from build123d import *

# Parameters (mm, degrees)
F0_R     = 11.2
F1_DEPTH = 7


with BuildPart() as f1:
    # F0 (on Top) → F1 (new body)
    with BuildSketch(Plane.XY):
        with BuildLine():
            Line((-21.939748, 4.555207), (-12.792678, 3.253825))
            ThreePointArc((-12.792678, 3.253825), (-11.283485, -6.850034), (-3.015751, -12.850885))
            Line((-3.015751, -12.850885), (-7.8557, -22.943517))
            Line((-7.8557, -22.943517), (-9.711457, -26.813285))
            Line((-9.711457, -26.813285), (-11.121781, -27.627536))
            Line((-11.121781, -27.627536), (-20.063522, -32.790052))
            Line((-20.063522, -32.790052), (-27.45722, -32.629778))
            Line((-27.45722, -32.629778), (-35.012019, -31.040825))
            Line((-35.012019, -31.040825), (-33.880058, -33.001439))
            Line((-33.880058, -33.001439), (-26.171613, -34.856514))
            Line((-26.171613, -34.856514), (-18.97682, -34.672275))
            Line((-18.97682, -34.672275), (-7.830637, -28.237023))
            Line((-7.830637, -28.237023), (-6.368866, -27.393069))
            Line((-6.368866, -27.393069), (-4.491412, -23.347324))
            Line((-4.491412, -23.347324), (0.218357, -13.198194))
            Line((0.218357, -13.198194), (3.914865, -22.392298))
            Line((3.914865, -22.392298), (5.384581, -26.047835))
            Line((5.384581, -26.047835), (6.257514, -26.551823))
            Line((6.257514, -26.551823), (18.746148, -33.762139))
            Line((18.746148, -33.762139), (24.941822, -34.300735))
            Line((24.941822, -34.300735), (33.179322, -33.454726))
            Line((33.179322, -33.454726), (34.46769, -31.223206))
            Line((34.46769, -31.223206), (26.169356, -32.174584))
            Line((26.169356, -32.174584), (19.596018, -31.214334))
            Line((19.596018, -31.214334), (9.226481, -25.227478))
            Line((9.226481, -25.227478), (8.427354, -24.766103))
            Line((8.427354, -24.766103), (7.024949, -21.277983))
            Line((7.024949, -21.277983), (3.578444, -12.705697))
            ThreePointArc((3.578444, -12.705697), (11.574046, -6.346768), (12.637068, 3.813725))
            Line((12.637068, 3.813725), (23.797519, 4.668523))
            Line((23.797519, 4.668523), (28.076715, 4.996274))
            Line((28.076715, 4.996274), (29.487039, 4.182023))
            Line((29.487039, 4.182023), (38.428779, -0.980493))
            Line((38.428779, -0.980493), (41.986827, -7.46376))
            Line((41.986827, -7.46376), (44.388153, -14.800885))
            Line((44.388153, -14.800885), (45.520113, -12.840272))
            Line((45.520113, -12.840272), (43.272433, -5.237025))
            Line((43.272433, -5.237025), (39.515481, 0.901729))
            Line((39.515481, 0.901729), (28.369297, 7.336981))
            Line((28.369297, 7.336981), (26.907526, 8.180935))
            Line((26.907526, 8.180935), (22.465082, 7.783985))
            Line((22.465082, 7.783985), (11.320793, 6.788199))
            Line((11.320793, 6.788199), (17.434867, 14.586522))
            Line((17.434867, 14.586522), (19.865796, 17.687101))
            Line((19.865796, 17.687101), (19.865796, 18.695077))
            Line((19.865796, 18.695077), (19.865796, 33.11571))
            Line((19.865796, 33.11571), (17.234397, 38.750619))
            Line((17.234397, 38.750619), (12.382981, 45.461498))
            Line((12.382981, 45.461498), (9.806245, 45.461498))
            Line((9.806245, 45.461498), (14.77933, 38.750619))
            Line((14.77933, 38.750619), (17.234397, 32.577816))
            Line((17.234397, 32.577816), (17.234397, 20.604106))
            Line((17.234397, 20.604106), (17.234397, 19.681354))
            Line((17.234397, 19.681354), (14.9148, 16.722776))
            Line((14.9148, 16.722776), (9.214235, 9.451872))
            ThreePointArc((9.214235, 9.451872), (-0.290561, 13.196802), (-9.621317, 9.03716))
            Line((-9.621317, 9.03716), (-15.941819, 18.274994))
            Line((-15.941819, 18.274994), (-18.365257, 21.817012))
            Line((-18.365257, 21.817012), (-18.365257, 23.445513))
            Line((-18.365257, 23.445513), (-18.365257, 33.770546))
            Line((-18.365257, 33.770546), (-14.529607, 40.093539))
            Line((-14.529607, 40.093539), (-9.376134, 45.84171))
            Line((-9.376134, 45.84171), (-11.640055, 45.84171))
            Line((-11.640055, 45.84171), (-17.10082, 40.093539))
            Line((-17.10082, 40.093539), (-20.538661, 33.770546))
            Line((-20.538661, 33.770546), (-20.538661, 20.900042))
            Line((-20.538661, 20.900042), (-20.538661, 19.212134))
            Line((-20.538661, 19.212134), (-17.97367, 15.563339))
            Line((-17.97367, 15.563339), (-11.53915, 6.409994))
            Line((-11.53915, 6.409994), (-21.349732, 7.805776))
            Line((-21.349732, 7.805776), (-25.250377, 8.360733))
            Line((-25.250377, 8.360733), (-26.12331, 7.856745))
            Line((-26.12331, 7.856745), (-38.611944, 0.646429))
            Line((-38.611944, 0.646429), (-42.176219, -4.449884))
            Line((-42.176219, -4.449884), (-45.562303, -12.006773))
            Line((-45.562303, -12.006773), (-44.273935, -14.238292))
            Line((-44.273935, -14.238292), (-40.948685, -6.576035))
            Line((-40.948685, -6.576035), (-36.830415, -1.363483))
            Line((-36.830415, -1.363483), (-26.460878, 4.623372))
            Line((-26.460878, 4.623372), (-25.661751, 5.084748))
            Line((-25.661751, 5.084748), (-21.939748, 4.555207))
        make_face()
        Circle(F0_R, mode=Mode.SUBTRACT)
        with BuildLine():
            Line((-9.711457, -26.813285), (-7.8557, -22.943517))
            ThreePointArc((-7.8557, -22.943517), (-12.025565, -21.787106), (-15.940622, -19.943903))
            ThreePointArc((-15.940622, -19.943903), (-16.27639, -12.118209), (-20.987711, -5.860599))
            ThreePointArc((-20.987711, -5.860599), (-23.219885, -4.563891), (-25.661751, -3.726428))
            ThreePointArc((-25.661751, -3.726428), (-41.175768, -20.890944), (-18.369131, -24.78487))
            ThreePointArc((-18.369131, -24.78487), (-14.840432, -26.448342), (-11.121781, -27.627536))
            Line((-11.121781, -27.627536), (-9.711457, -26.813285))
        make_face()
        with Locations((-28.702531, -16.571414)):
            Circle(F0_R, mode=Mode.SUBTRACT)
        with BuildLine():
            Line((-6.368866, -27.393069), (-7.830637, -28.237023))
            ThreePointArc((-7.830637, -28.237023), (-0.682852, -28.261424), (6.257514, -26.551823))
            Line((6.257514, -26.551823), (5.384581, -26.047835))
            Line((5.384581, -26.047835), (3.914865, -22.392298))
            ThreePointArc((3.914865, -22.392298), (-0.248488, -23.220008), (-4.491412, -23.347324))
            Line((-4.491412, -23.347324), (-6.368866, -27.393069))
        make_face()
        with BuildLine():
            Line((8.427354, -24.766103), (9.226481, -25.227478))
            ThreePointArc((9.226481, -25.227478), (12.8176, -23.040102), (16.058057, -20.360514))
            ThreePointArc((16.058057, -20.360514), (38.679972, -25.213789), (30.648892, -3.515699))
            ThreePointArc((30.648892, -3.515699), (30.325152, 0.37198), (29.487039, 4.182023))
            Line((29.487039, 4.182023), (28.076715, 4.996274))
            Line((28.076715, 4.996274), (23.797519, 4.668523))
            ThreePointArc((23.797519, 4.668523), (24.88097, 0.479108), (25.242237, -3.833032))
            ThreePointArc((25.242237, -3.833032), (18.632872, -8.036663), (15.569283, -15.245592))
            ThreePointArc((15.569283, -15.245592), (11.608949, -18.703471), (7.024949, -21.277983))
            Line((7.024949, -21.277983), (8.427354, -24.766103))
        make_face()
        with Locations((28.702531, -16.571414)):
            Circle(F0_R, mode=Mode.SUBTRACT)
        with BuildLine():
            ThreePointArc((28.369297, 7.336981), (24.816537, 13.539344), (19.865796, 18.695077))
            Line((19.865796, 18.695077), (19.865796, 17.687101))
            Line((19.865796, 17.687101), (17.434867, 14.586522))
            ThreePointArc((17.434867, 14.586522), (20.233361, 11.394807), (22.465082, 7.783985))
            Line((22.465082, 7.783985), (26.907526, 8.180935))
            Line((26.907526, 8.180935), (28.369297, 7.336981))
        make_face()
        with BuildLine():
            ThreePointArc((-12.279761, 28.300569), (-15.48472, 26.076362), (-18.365257, 23.445513))
            Line((-18.365257, 23.445513), (-18.365257, 21.817012))
            Line((-18.365257, 21.817012), (-15.941819, 18.274994))
            ThreePointArc((-15.941819, 18.274994), (-12.855404, 21.307998), (-9.301616, 23.776935))
            ThreePointArc((-9.301616, 23.776935), (-2.356482, 20.154872), (5.418428, 21.10619))
            ThreePointArc((5.418428, 21.10619), (10.393206, 19.40538), (14.9148, 16.722776))
            Line((14.9148, 16.722776), (17.234397, 19.681354))
            Line((17.234397, 19.681354), (17.234397, 20.604106))
            ThreePointArc((17.234397, 20.604106), (13.544514, 22.620419), (9.603694, 24.086942))
            ThreePointArc((9.603694, 24.086942), (2.495796, 46.104733), (-12.279761, 28.300569))
        make_face()
        with Locations((0, 33.142827)):
            Circle(F0_R, mode=Mode.SUBTRACT)
        with BuildLine():
            ThreePointArc((-20.538661, 20.900042), (-24.133685, 14.722079), (-26.12331, 7.856745))
            Line((-26.12331, 7.856745), (-25.250377, 8.360733))
            Line((-25.250377, 8.360733), (-21.349732, 7.805776))
            ThreePointArc((-21.349732, 7.805776), (-19.984873, 11.825201), (-17.97367, 15.563339))
            Line((-17.97367, 15.563339), (-20.538661, 19.212134))
            Line((-20.538661, 19.212134), (-20.538661, 20.900042))
        make_face()
        with BuildLine():
            ThreePointArc((-20.987711, -5.860599), (-22.002156, -0.701909), (-21.939748, 4.555207))
            Line((-21.939748, 4.555207), (-25.661751, 5.084748))
            Line((-25.661751, 5.084748), (-26.460878, 4.623372))
            ThreePointArc((-26.460878, 4.623372), (-26.362114, 0.419684), (-25.661751, -3.726428))
            ThreePointArc((-25.661751, -3.726428), (-23.219885, -4.563891), (-20.987711, -5.860599))
        make_face()
    extrude(amount=F1_DEPTH)


solid = f1.part
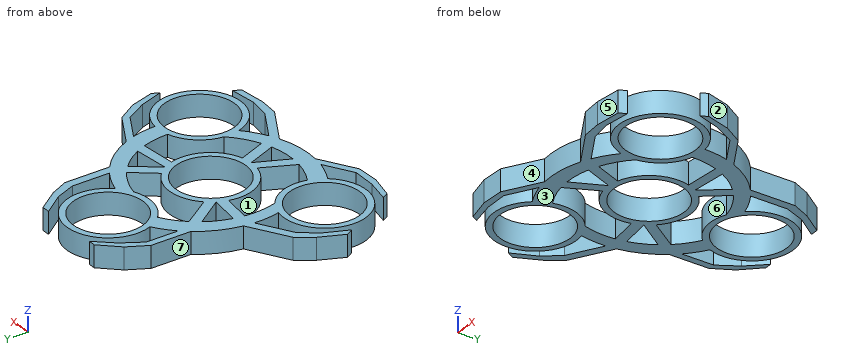
Could you check a few things on this model? Use its own coordinates, in mm. Face numbers are marked on the shaded views. A direction names the side the tool comes from. Coordinates: 2 decimals unless noted, no trailing zeros. Order: outer loops, then holes, each group sorted by start corner. A loop starts at its lowest first (then second) coordinate and runs counter-clockwise, first axis right, second up. Notation, with made-up numbers: (45.25, -17.75) - (54.25, -17.75) arc R9 ccw to (54.25, -7.75) - close; hole circle Ø8 at (47.5, -2). An arc over 180 degrees is marked (long way). Answer in a Markdown table with one row per item. Add a question column.
(1) I need wall thicknesses on L1, parallel to Y at x = -1.5, z = 4.75; L2, parallel to X at y = 34, z = 2.5; L3, parallel to Y at x = -12, z = 5. Which ranges of each line are inside material? Lowest first, please.
(2) On a 3-axis mill with a long thin cutter (end or side, diameter ignored), from which of +Z, -Z, +X, -X, +Y, -Y can I reach the whole of each face in a straight line? I mean the marked faces 4, 5, 6 and 7. Say none if no direction works.
(3) If we mould it in two halves opening along X, with no side actions, what happens to the marked faces 1, 2 and 3? For each: released by +X, released by -X, zero draft, split by the parting line, or undercut.
(4) If we section it at B-B, the plane x = -1: Please give me the cut outline in (y, z).
(5) If we section it at C-C, the plane z = 1: State how many separate pieces and enclosed holes the cut face has, then the cut area to 3 significant figures.
(6) Will these pins go through, and if not, where does the flat tip stop? pin 1 (2 mm diameter, centred on y = 25.5, z = 5, fed in from -X); pin 2 (2 mm diameter, centred on y = 26, z = 4.5, fed in from +X); pin 3 (1 mm diameter, centred on x = -29.5, z = 2.5, fed in from +Y).
(7) If we section it at D-D, the plane y = 27: Please give me the cut outline in (x, z), then the cut area to 3 significant figures.
(8) If we section it at A-A, the plane y = 36.5: Please give me the cut outline in (x, z) (3 decimals).
Results are:
| question | item | result |
|---|---|---|
| 1 | L1 | y = -28.35 to -23.33, -16.9 to -11.1, 11.1 to 13.11, 20.03 to 22.04, 44.24 to 46.26 |
| 1 | L2 | x = -20.41 to -18.23, -13.17 to -11.17, 11.17 to 13.17, 16.67 to 19.45 |
| 1 | L3 | y = -30.64 to -28.13, -27.4 to -21.8, -5.5 to 6.48, 7.07 to 12.51, 21.99 to 38.64, 42.92 to 45.46 |
| 2 | face 4 | +Z, -Z, -Y |
| 2 | face 5 | +Z, -Z, +X, -Y |
| 2 | face 6 | +Z, -Z |
| 2 | face 7 | +Z, -Z, -X, +Y |
| 3 | face 1 | undercut |
| 3 | face 2 | released by +X |
| 3 | face 3 | zero draft |
| 4 | outline | (-28.3, 0) - (-23.29, 0) - (-23.29, 7) - (-28.3, 7) - close; (-15.82, 0) - (-11.16, 0) - (-11.16, 7) - (-15.82, 7) - close; (11.16, 0) - (13.16, 0) - (13.16, 7) - (11.16, 7) - close; (19.98, 0) - (21.99, 0) - (21.99, 7) - (19.98, 7) - close; (44.3, 0) - (46.3, 0) - (46.3, 7) - (44.3, 7) - close |
| 5 | separate pieces | 1 |
| 5 | enclosed holes | 10 |
| 5 | area | 1,690 mm2 |
| 6 | pin 1 | stops at x = -20.54 |
| 6 | pin 2 | stops at x = 19.87 |
| 6 | pin 3 | stops at y = 6.2 |
| 7 | outline | (-20.54, 0) - (-18.37, 0) - (-18.37, 7) - (-20.54, 7) - close; (-14.26, 0) - (-9.37, 0) - (-9.37, 7) - (-14.26, 7) - close; (9.37, 0) - (11.68, 0) - (11.68, 7) - (9.37, 7) - close; (17.23, 0) - (19.87, 0) - (19.87, 7) - (17.23, 7) - close |
| 7 | area | 84.1 mm2 |
| 8 | outline | (-19.055, 0) - (-16.71, 0) - (-16.71, 7) - (-19.055, 7) - close; (-12.766, 0) - (-10.685, 0) - (-10.685, 7) - (-12.766, 7) - close; (10.685, 0) - (12.766, 0) - (12.766, 7) - (10.685, 7) - close; (15.674, 0) - (18.285, 0) - (18.285, 7) - (15.674, 7) - close |
